Read the model definition and answer for the solid it produces. Units are mm, in the model's axes. A direction names the side the tool comes from. Coordinates: 2 decimals unless noted, no trailing zeros. Loops run counter-clockwise (first coordinate to the right, second up) from the corner with the lowest first, then second, coordinate; pieces in that order, holes last. Notation, with made-up numbers: (69, 64.5) -> (122, 64.5) arc R23 ccw to (122, 77.5) -> close; hole circle Ø11 at (35, 58). An arc over 180 degrees is marked (long way). Answer in a Markdown table with one row per item.
```python
from build123d import *

# Parameters (mm, degrees)
SK_BOARD_W              = 50
SK_BOARD_H              = 50
EX_BOARD_DEPTH          = 1.6
SK_MOUNTHOLES_4X_R      = 1.5
CUT_MOUNTHOLES_4X_DEPTH = 1.6
SK_COMPONENTS_W         = 44
SK_COMPONENTS_H         = 38
EX_COMPONENTS_DEPTH     = 9.3
SK_PINS_W               = 40
SK_PINS_H               = 40
EX_PINS_DEPTH           = 1.6


with BuildPart() as part:
    # SK_Board → EX_Board (new body)
    with BuildSketch(Plane(origin=(0, 0, 0), x_dir=(1, 0, 0), z_dir=(0, 1, 0))):
        Rectangle(SK_BOARD_W, SK_BOARD_H)
    extrude(amount=EX_BOARD_DEPTH)

    # SK_MountHoles_4x → CUT_MountHoles_4x (cut)
    with BuildSketch(Plane(origin=(0, 0, 0), x_dir=(1, 0, 0), z_dir=(0, 1, 0))):
        with Locations(Location((22.5, -22.5, 0), (0, 0, 270))):
            Circle(SK_MOUNTHOLES_4X_R)
        with Locations(Location((-22.5, -22.5, 0), (0, 0, 270))):
            Circle(SK_MOUNTHOLES_4X_R)
        with Locations(Location((22.5, 22.5, 0), (0, 0, 270))):
            Circle(SK_MOUNTHOLES_4X_R)
        with Locations(Location((-22.5, 22.5, 0), (0, 0, 270))):
            Circle(SK_MOUNTHOLES_4X_R)
    extrude(amount=CUT_MOUNTHOLES_4X_DEPTH, mode=Mode.SUBTRACT)

    # SK_Components → EX_Components (add)
    with BuildSketch(Plane(origin=(0, 1.6, 0), x_dir=(1, 0, 0), z_dir=(0, 1, 0))):
        Rectangle(SK_COMPONENTS_W, SK_COMPONENTS_H)
    extrude(amount=EX_COMPONENTS_DEPTH)

    # SK_Pins → EX_Pins (add)
    with BuildSketch(Plane(origin=(0, 0, 0), x_dir=(1, 0, 0), z_dir=(0, 1, 0))):
        Rectangle(SK_PINS_W, SK_PINS_H)
    extrude(amount=-EX_PINS_DEPTH)


solid = part.part
```
1. A cutting plane is placed at C-C on z = 9. Give the vertices of the cut face in (x, y), and give its area (3 significant figures).
A:
| item | result |
|---|---|
| outline | (-25, 0) -> (-20, 0) -> (-20, -1.6) -> (20, -1.6) -> (20, 0) -> (25, 0) -> (25, 1.6) -> (22, 1.6) -> (22, 10.9) -> (-22, 10.9) -> (-22, 1.6) -> (-25, 1.6) -> close |
| area | 553 mm2 |
2. The mould has two halves that part along X. Classify faces 5 (the flat face through (0, 1, 25)), 6 (the cylindrical face through (23.51, 0.79, 21.39)), 7 (the flat face through (20, -1, 0)), 8 (the cylindrical face through (23.51, 0.79, -23.61)): pulls with the +X half, pulls with the -X half, needs draft (parallel to the pull), parting line crosses it, or undercut.
A:
| item | result |
|---|---|
| face 5 | needs draft |
| face 6 | undercut |
| face 7 | pulls with the +X half |
| face 8 | undercut |
3. Given pin 1 Ø4.5 at (y, z) = (6, 0.5) entering from -X; pin 2 Ø7.5 at (y, z) = (5.5, 4) entering from +X; pin 3 Ø0.5 at (x, y) = (-8.5, -1) entering from -Z, each flat-ended and moving along its own axis, determine where each tip first touches the part or whether it passes through.
A:
| item | result |
|---|---|
| pin 1 | stops at x = -22 |
| pin 2 | stops at x = 22 |
| pin 3 | stops at z = -20 |
4. A cutting plane is placed at A-A on z = -22.5. Give the vertices of the cut face in (x, y), and give its area (3 significant figures).
A:
| item | result |
|---|---|
| outline | (-25, 0) -> (-24, 0) -> (-24, 1.6) -> (-25, 1.6) -> close; (-21, 0) -> (21, 0) -> (21, 1.6) -> (-21, 1.6) -> close; (24, 0) -> (25, 0) -> (25, 1.6) -> (24, 1.6) -> close |
| area | 70.4 mm2 |
5. A cutting plane is placed at B-B on x = -16. Give the vertices of the cut face in (y, z).
A:
| item | result |
|---|---|
| outline | (-1.6, -20) -> (0, -20) -> (0, -25) -> (1.6, -25) -> (1.6, -19) -> (10.9, -19) -> (10.9, 19) -> (1.6, 19) -> (1.6, 25) -> (0, 25) -> (0, 20) -> (-1.6, 20) -> close |
6. A tool of negligible diameter and unlimited length cuts with its end or side. For faces 1 (the flat face through (0, -1, -20)), 2 (the flat face through (0, 6, -19)), 3 (the flat face through (0, -1, 20)), 4 (the flat face through (0, 6, 19)), from which of +Z, -Z, +X, -X, +Y, -Y can it reach the whole face along a straight path? Write none if from no direction.
A:
| item | result |
|---|---|
| face 1 | -Z, +X, -X, -Y |
| face 2 | -Z, +X, -X, +Y |
| face 3 | +Z, +X, -X, -Y |
| face 4 | +Z, +X, -X, +Y |
7. Find the intervals of material crossed by probe 1 along X at (y, z) = (0.85, -22.5); probe 2 along Z at (x, y) = (12.5, 3.75); probe 3 along X at (y, z) = (7, 15.5), in increasing order.
A:
| item | result |
|---|---|
| probe 1 | x = -25 to -24, -21 to 21, 24 to 25 |
| probe 2 | z = -19 to 19 |
| probe 3 | x = -22 to 22 |
8. A cutting plane is placed at D-D on y = 9.25. Give the vertices of the cut face in (x, z), and give its area (3 significant figures).
A:
| item | result |
|---|---|
| outline | (-22, -19) -> (22, -19) -> (22, 19) -> (-22, 19) -> close |
| area | 1,670 mm2 |
